Could you check a few things on this model? Use its own coordinates, in mm. A direction names the side the tool comes from. Give positions to 0.01 mm unless a question says otherwise; leave off trailing zeros. Loops run counter-clockwise (first coordinate to the right, second up) from the corner with the lowest first, then second, coordinate; pieces in that order, holes last. Notation, with made-up numbers: M 44.5,58 L 77.5,58 A28 ccw 77.5,79 Z; hole C 43,55 d2. An arc over 180 degrees is marked long. Use a Markdown table: item, result. Add a question column.
1) Suppose I cut it at D-D on y = 0.9. List the corners of the cut face in (x, z) for me.
2) Will these pins go through, and if not, where does the flat tip stop? pin 1 Ø0.8 at (x, y) = (-9.5, 0.5) entering from +Z; pin 2 Ø0.8 at (x, y) = (-9, 0.5) entering from -Z.
3) Suppose I cut it at A-A on x = -5. List the corners of the cut face in (y, z) for me, and give its area (3 significant figures).
4) We'd pull the mould along Z, two halves only. Please class faces 1 (the cylindrical face through (-0.176, 0.74, -16.339)), 2 (the flat face through (-21.5, 1, 0)), 3 (the flat face through (-12, 1, -12)), 4 (the cylindrical face through (3, 1, 1)): +Z half, -Z half, draft (parallel to the pull), parting line (faces both ways), or undercut.
5) Suppose I cut it at B-B on z = 1. List the corners of the cut face in (x, y) for me, and give its area (3 significant figures).
6) If I drill on line 1 along Z through (x, y) = (-19.3, 1.2); line 2 along Z through (x, y) = (0, 0.35); line 3 along X through (y, z) = (0.9, -15), over which ranges is the centre line in solid material (lowest first)? Write a range as [from, to].
7) Suppose I cut it at C-C on x = -19.3. List the corners of the cut face in (y, z) for me.
8) Which directions (+Z, -Z, +X, -X, +Y, -Y) give clear straight access to the entire face, cutting with the end or side of a thin tool? Please do faces 5 (the flat face through (-2.5, 1, -14)), 6 (the flat face through (-10, 1, 4)), 7 (the flat face through (2.5, 1, 14)), 8 (the flat face through (-2.5, 1, 13)), 9 (the flat face through (10, 1, -12)).
```python
from build123d import *

# Parameters (mm, degrees)
SKETCH1_W           = 35
SKETCH1_H           = 24
SKETCH1_R           = 3
SKETCH1_R_2         = 2.5
SKETCH1_R_3         = 1.35
SKETCH1_W_2         = 4
BOSS_EXTRUDE1_DEPTH = 1.5
CUT_EXTRUDE1_DEPTH  = 10


with BuildPart() as part:
    # Sketch1 → Boss-Extrude1 (new body)
    with BuildSketch(Plane(origin=(0, 0, 0), x_dir=(1, 0, 0), z_dir=(0, 1, 0))):
        Rectangle(SKETCH1_W, SKETCH1_H)
        with Locations((0, -1)):
            Circle(SKETCH1_R, mode=Mode.SUBTRACT)
        with BuildLine():
            Line((2.5, -12), (-2.5, -12))
            Line((-2.5, -12), (-2.5, -15))
            ThreePointArc((-2.5, -15), (0, -12.5), (2.5, -15))
            Line((2.5, -15), (2.5, -12))
        make_face()
        with Locations((0, -15)):
            Circle(SKETCH1_R_2)
        with Locations((0, -15)):
            Circle(SKETCH1_R_3, mode=Mode.SUBTRACT)
        with BuildLine():
            Line((-2.5, 15), (-2.5, 12))
            Line((-2.5, 12), (2.5, 12))
            Line((2.5, 12), (2.5, 15))
            ThreePointArc((2.5, 15), (0, 12.5), (-2.5, 15))
        make_face()
        with Locations((0, 15)):
            Circle(SKETCH1_R_2)
        with Locations((0, 15)):
            Circle(SKETCH1_R_3, mode=Mode.SUBTRACT)
        with Locations((-19.5, 0)):
            Rectangle(SKETCH1_W_2, SKETCH1_H)
        with Locations((-19.3, 7.75)):
            Circle(SKETCH1_R_3, mode=Mode.SUBTRACT)
        with Locations((-19.3, -9.75)):
            Circle(SKETCH1_R_3, mode=Mode.SUBTRACT)
    extrude(amount=BOSS_EXTRUDE1_DEPTH)

    # Sketch2 → Cut-Extrude1 (cut)
    with BuildSketch(Plane(origin=(0, 1.5, 0), x_dir=(1, 0, 0), z_dir=(0, 1, 0))):
        with BuildLine():
            Line((0, 2), (-20, 2))
            Line((-20, 2), (-20, -4))
            Line((-20, -4), (0, -4))
            ThreePointArc((0, -4), (3, -1), (0, 2))
        make_face()
    extrude(amount=-CUT_EXTRUDE1_DEPTH, mode=Mode.SUBTRACT)


solid = part.part
```
Answer block:
| question | item | result |
|---|---|---|
| 1 | outline | M -21.5,-12 L -2.5,-12 L -2.5,-15 A2.5 ccw 2.5,-15 L 2.5,-12 L 17.5,-12 L 17.5,12 L 2.5,12 L 2.5,15 A2.5 ccw -2.5,15 L -2.5,12 L -21.5,12 Z; hole C -19.3,-7.75 d2.7; hole C -19.3,9.75 d2.7; hole M -20,-2 L 0,-2 A3 ccw 0,4 L -20,4 Z; hole C 0,-15 d2.7; hole C 0,15 d2.7 |
| 2 | pin 1 | stops at z = 12 |
| 2 | pin 2 | stops at z = -12 |
| 3 | outline | M 0,-12 L 1.5,-12 L 1.5,-2 L 0,-2 Z; M 0,4 L 1.5,4 L 1.5,12 L 0,12 Z |
| 3 | area | 27.0 mm^2 |
| 4 | face 1 | undercut |
| 4 | face 2 | draft |
| 4 | face 3 | -Z half |
| 4 | face 4 | undercut |
| 5 | outline | M -21.5,0 L -20,0 L -20,1.5 L -21.5,1.5 Z; M 3,0 L 17.5,0 L 17.5,1.5 L 3,1.5 Z |
| 5 | area | 24.0 mm^2 |
| 6 | line 1 | z = [-12, -9.1], [-6.4, -2], [4, 8.4], [11.1, 12] |
| 6 | line 2 | z = [-17.5, -16.35], [-13.65, -2], [4, 13.65], [16.35, 17.5] |
| 6 | line 3 | x = [-2.5, -1.35], [1.35, 2.5] |
| 7 | outline | M 0,-12 L 1.5,-12 L 1.5,-9.1 L 0,-9.1 Z; M 0,-6.4 L 1.5,-6.4 L 1.5,-2 L 0,-2 Z; M 0,4 L 1.5,4 L 1.5,8.4 L 0,8.4 Z; M 0,11.1 L 1.5,11.1 L 1.5,12 L 0,12 Z |
| 8 | face 5 | -Z, -X, +Y, -Y |
| 8 | face 6 | +Y, -Y |
| 8 | face 7 | +Z, +X, +Y, -Y |
| 8 | face 8 | +Z, -X, +Y, -Y |
| 8 | face 9 | -Z, +X, +Y, -Y |
